Verification items for the finished model (mm, model axes). Face numbers are marked on the shaded views. A direction names the side the tool comes from. Give positions to 0.01 mm unless a question says otherwise; leave off trailing zeros. Loops run counter-clockwise (first coordinate to the right, second up) from the corner with the lowest first, then second, coordinate; pieces in that order, holes last. Notation, with made-up numbers: (-1.75, 58.5) - (28.25, 58.5) arc R24 ccw to (28.25, 77.5) - close; hole circle Ø9 at (36, 27.25). An arc over 180 degrees is marked (long way). One line per item, written item: value. Start each with the question number.
1. Sectioned sample at B-B (y = 52). Record the cut outline in (x, z), plus the area to 3 significant figures.
2. Access from +Z, -Z, +X, -X, +Y, -Y to the whole of each face (thin tool, end or side, straight path). Record for the marked faces 5 and 6.
3. Sectioned sample at D-D (x = -19). Record the cut outline in (y, z), plus the area to 3 significant figures.
4. Mould release check, pull along X, two halves, no side actions. Record for the marked faces 1, 2, 3 and 4: pulls with the +X half, pulls with the -X half, needs draft (parallel to the pull), parting line crosses it, or undercut.
5. Sectioned sample at C-C (z = -13). Record the cut outline in (x, y).
6. Scan lines: L1, parallel to X at y = 38.5, z = -22.5; L2, parallel to Z at x = 29, y = 10. Record each from-to range of solid material in increasing order. Write a range as [from, to].
7. Sectioned sample at A-A (z = -21.5). Record the cut outline in (x, y).
8. Gauge pin test, flat end, axial feed: pin 1 (10 mm diameter, centred on x = 29, y = 9.5, fed in from -Z). Record the tip position at first contact, or that the pin passes through.
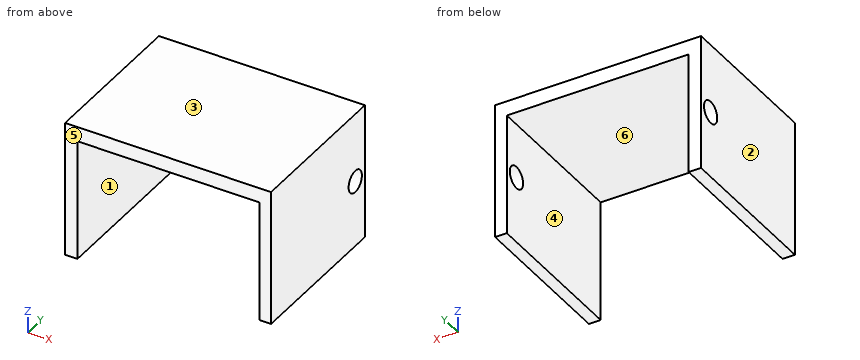
from build123d import *

# Parameters (mm, degrees)
SALIENTE_EXTRUIR2_DEPTH = 60
CROQUIS4_R              = 4.23503961
CORTAR_EXTRUIR1_DEPTH   = 110


with BuildPart() as part:
    # Croquis3 → Saliente-Extruir2 (new body)
    with BuildSketch(Plane(origin=(0, 0, 0), x_dir=(1, 0, 0), z_dir=(0, 1, 0))):
        Polygon((-33.38838539, 0), (-33.38838539, 39.424440528), (-28.644268776, 39.424440528), (-28.644268776, 0), (-28.644268776, -7.338994669), (41.387928863, -7.338994669), (41.387928863, 39.424440528), (45.906135162, 39.424440528), (45.906135162, -12.986752543), (-33.38838539, -12.986752543), align=None)
    extrude(amount=SALIENTE_EXTRUIR2_DEPTH)

    # Croquis4 → Cortar-Extruir1 (cut)
    with BuildSketch(Plane.ZY.offset(33.38838539)):
        with Locations((-13.763852604, 53.844361948)):
            Circle(CROQUIS4_R)
    extrude(amount=-CORTAR_EXTRUIR1_DEPTH, mode=Mode.SUBTRACT)


solid = part.part
Results are:
1. outline: (-33.39, -39.42) - (-28.64, -39.42) - (-28.64, -17.58) - (-33.39, -17.58) - close; (-33.39, -9.95) - (-28.64, -9.95) - (-28.64, 7.34) - (41.39, 7.34) - (41.39, -9.95) - (45.91, -9.95) - (45.91, 12.99) - (-33.39, 12.99) - close; (41.39, -39.42) - (45.91, -39.42) - (45.91, -17.58) - (41.39, -17.58) - close
1. area: 810 mm^2
2. face 5: +Z, -Z, +X, -X, -Y
2. face 6: -Z, +Y, -Y
3. outline: (0, 7.34) - (60, 7.34) - (60, 12.99) - (0, 12.99) - close
3. area: 339 mm^2
4. face 1: undercut
4. face 2: pulls with the -X half
4. face 3: needs draft
4. face 4: undercut
5. outline: (-33.39, 0) - (-28.64, 0) - (-28.64, 49.68) - (-33.39, 49.68) - close; (-33.39, 58.01) - (-28.64, 58.01) - (-28.64, 60) - (-33.39, 60) - close; (41.39, 0) - (45.91, 0) - (45.91, 49.68) - (41.39, 49.68) - close; (41.39, 58.01) - (45.91, 58.01) - (45.91, 60) - (41.39, 60) - close
6. L1: x = [-33.39, -28.64], [41.39, 45.91]
6. L2: z = [7.34, 12.99]
7. outline: (-33.39, 0) - (-28.64, 0) - (-28.64, 60) - (-33.39, 60) - close; (41.39, 0) - (45.91, 0) - (45.91, 60) - (41.39, 60) - close
8. pin 1: stops at z = 7.34
